```python
from build123d import *

# Parameters (mm, degrees)
SKETCH1_W           = 45
SKETCH1_H           = 37.5
BOSS_EXTRUDE1_DEPTH = 2
SKETCH2_W           = 40
SKETCH2_H           = 13
BOSS_EXTRUDE2_DEPTH = 7
BOSS_EXTRUDE3_DEPTH = 15
FILLET1_R           = 1
SKETCH4_W           = 10
SKETCH4_H           = 8
CUT_EXTRUDE1_DEPTH  = 5
SKETCH5_W           = 41
SKETCH5_H           = 14
CUT_EXTRUDE2_DEPTH  = 7
SKETCH6_W           = 11
SKETCH6_H           = 20
BOSS_EXTRUDE5_DEPTH = 12
SKETCH7_W           = 9
SKETCH7_H           = 9
CUT_EXTRUDE3_DEPTH  = 12


with BuildPart() as part:
    # Sketch1 → Boss-Extrude1 (new body)
    with BuildSketch(Plane.XY):
        Rectangle(SKETCH1_W, SKETCH1_H)
    extrude(amount=BOSS_EXTRUDE1_DEPTH)

    # Sketch2 → Boss-Extrude2 (add)
    with BuildSketch(Plane.XY.offset(2)):
        with Locations((0, -11.25)):
            Rectangle(SKETCH2_W, SKETCH2_H)
    extrude(amount=BOSS_EXTRUDE2_DEPTH)

    # Sketch3 → Boss-Extrude3 (add)
    with BuildSketch(Plane.XY.offset(9)):
        Polygon((-5, -7.25), (-5, -5.25), (-15, -5.25), (-15, -17.25), (-5, -17.25), (-5, -15.25), (5, -15.25), (5, -17.25), (15, -17.25), (15, -5.25), (5, -5.25), (5, -7.25), align=None)
    extrude(amount=BOSS_EXTRUDE3_DEPTH)

    # Fillet1
    fillet1_edges = [part.edges().sort_by_distance(p)[0] for p in [
        (5, -5.25, 16.5),
        (-5, -5.25, 16.5),
        (-15, -5.25, 16.5),
        (-15, -17.25, 16.5),
        (-5, -17.25, 16.5),
        (5, -17.25, 16.5),
        (15, -17.25, 16.5),
        (15, -5.25, 16.5),
    ]]
    fillet(fillet1_edges, radius=FILLET1_R)

    # Sketch4 → Cut-Extrude1 (cut)
    with BuildSketch(Plane.XY.offset(24)):
        with BuildLine():
            Line((-5.5, -14.75), (-5.5, -7.75))
            Line((-5.5, -7.75), (-5.5, -6.25))
            ThreePointArc((-5.5, -6.25), (-5.646446609, -5.896446609), (-6, -5.75))
            Line((-6, -5.75), (-14, -5.75))
            ThreePointArc((-14, -5.75), (-14.353553391, -5.896446609), (-14.5, -6.25))
            Line((-14.5, -6.25), (-14.5, -16.25))
            ThreePointArc((-14.5, -16.25), (-14.353553391, -16.603553391), (-14, -16.75))
            Line((-14, -16.75), (-6, -16.75))
            ThreePointArc((-6, -16.75), (-5.646446609, -16.603553391), (-5.5, -16.25))
            Line((-5.5, -16.25), (-5.5, -14.75))
        make_face()
        with BuildLine():
            Line((5.5, -7.75), (5.5, -14.75))
            Line((5.5, -14.75), (5.5, -16.25))
            ThreePointArc((5.5, -16.25), (5.646446609, -16.603553391), (6, -16.75))
            Line((6, -16.75), (14, -16.75))
            ThreePointArc((14, -16.75), (14.353553391, -16.603553391), (14.5, -16.25))
            Line((14.5, -16.25), (14.5, -6.25))
            ThreePointArc((14.5, -6.25), (14.353553391, -5.896446609), (14, -5.75))
            Line((14, -5.75), (6, -5.75))
            ThreePointArc((6, -5.75), (5.646446609, -5.896446609), (5.5, -6.25))
            Line((5.5, -6.25), (5.5, -7.75))
        make_face()
        with Locations((0, -11.25)):
            Rectangle(SKETCH4_W, SKETCH4_H)
    extrude(amount=-CUT_EXTRUDE1_DEPTH, mode=Mode.SUBTRACT)

    # Sketch5 → Cut-Extrude2 (cut)
    with BuildSketch(Plane.XY.offset(9)):
        with Locations((0, -11.25)):
            Rectangle(SKETCH5_W, SKETCH5_H)
        with BuildLine():
            Line((-14, -17.75), (-6, -17.75))
            ThreePointArc((-6, -17.75), (-4.939339828, -17.310660172), (-4.5, -16.25))
            Line((-4.5, -16.25), (-4.5, -15.75))
            Line((-4.5, -15.75), (4.5, -15.75))
            Line((4.5, -15.75), (4.5, -16.25))
            ThreePointArc((4.5, -16.25), (4.939339828, -17.310660172), (6, -17.75))
            Line((6, -17.75), (14, -17.75))
            ThreePointArc((14, -17.75), (15.060660172, -17.310660172), (15.5, -16.25))
            Line((15.5, -16.25), (15.5, -13.75))
            Line((15.5, -13.75), (17.5, -13.75))
            ThreePointArc((17.5, -13.75), (20, -11.25), (17.5, -8.75))
            Line((17.5, -8.75), (15.5, -8.75))
            Line((15.5, -8.75), (15.5, -6.25))
            ThreePointArc((15.5, -6.25), (15.060660172, -5.189339828), (14, -4.75))
            Line((14, -4.75), (6, -4.75))
            ThreePointArc((6, -4.75), (4.939339828, -5.189339828), (4.5, -6.25))
            Line((4.5, -6.25), (4.5, -6.75))
            Line((4.5, -6.75), (-4.5, -6.75))
            Line((-4.5, -6.75), (-4.5, -6.25))
            ThreePointArc((-4.5, -6.25), (-4.939339828, -5.189339828), (-6, -4.75))
            Line((-6, -4.75), (-14, -4.75))
            ThreePointArc((-14, -4.75), (-15.060660172, -5.189339828), (-15.5, -6.25))
            Line((-15.5, -6.25), (-15.5, -8.75))
            Line((-15.5, -8.75), (-17.5, -8.75))
            ThreePointArc((-17.5, -8.75), (-20, -11.25), (-17.5, -13.75))
            Line((-17.5, -13.75), (-15.5, -13.75))
            Line((-15.5, -13.75), (-15.5, -16.25))
            ThreePointArc((-15.5, -16.25), (-15.060660172, -17.310660172), (-14, -17.75))
        make_face(mode=Mode.SUBTRACT)
    extrude(amount=-CUT_EXTRUDE2_DEPTH, mode=Mode.SUBTRACT)

    # Sketch6 → Boss-Extrude5 (add)
    with BuildSketch(Plane(origin=(0, 0, 0), x_dir=(-1, 0, 0), z_dir=(0, 0, -1))):
        with Locations((-6, 8.25)):
            Rectangle(SKETCH6_W, SKETCH6_H)
        with Locations((6, 8.25)):
            Rectangle(SKETCH6_W, SKETCH6_H)
    extrude(amount=BOSS_EXTRUDE5_DEPTH)

    # Sketch7 → Cut-Extrude3 (cut)
    with BuildSketch(Plane(origin=(0, 18.25, 0), x_dir=(1, 0, 0), z_dir=(0, 1, 0))):
        with Locations((-6, 5.5)):
            Rectangle(SKETCH7_W, SKETCH7_H)
        with Locations((6, 5.5)):
            Rectangle(SKETCH7_W, SKETCH7_H)
    extrude(amount=-CUT_EXTRUDE3_DEPTH, mode=Mode.SUBTRACT)


solid = part.part
```
CAD build for the part. Positions are in the model's coordinates, mm. A direction names the side the tool comes from. Round coordinates to 2 decimals unless told otherwise and drop trailing zeros. Order: outer loops, then holes, each group sorted by start corner. A loop starts at its lowest first (then second) coordinate and runs counter-clockwise, first axis right, second up.
Q1. Slice it at B-B (z = 11.5). Write the cut outline in (x, y), and give its area (3 significant figures).
Q2. Wall check: L1, parallel to X at y = 10.5, z = -3.5; L2, parallel to X at y = -16, z = 10.5; L3, parallel to Z at x = 1, y = 5.5. Give the ranges that are in metal, low to high.
Q3. Which spindle directions (+Z, -Z, +X, -X, +Y, -Y) get a long thin tool onto all of the face, cutting with end or side? Do faces 1 (the cylindrical face through (-15.05, -5.18, 5.55)), 2 (the flat face through (-1, 18.25, -6)), 3 (the flat face through (15.5, -8, 6)), 4 (the cylindrical face through (15.05, -17.32, 5.55)), 5 (the flat face through (10, -16.75, 22)). Say none if no direction does.
Q4. Slice it at C-C (x = -9). Write the cut outline in (y, z), and give its area (3 significant figures).
Q5. Slice it at D-D (z = -2). Write the cut outline in (x, y).
Q6. Slice it at A-A (y = 8). Write the cut outline in (x, z).
Q7. Two-plate mould, pull along Z, no slides. Class faces 6 (the flat face through (10.5, 12, -5)), 7 (the flat face through (-10, -5.25, 16)), 8 (the flat face through (0, -11, 19)): pulls with the +Z half, pulls with the -Z half, needs draft (parallel to the pull), parting line crosses it, or undercut.
Q8. Drop flat-ended pins along their axis: pin 1 (10 mm diameter, centred on x = 6, y = 14.5, fed in from +Z); pin 2 (0.8 mm diameter, centred on y = -15.5, z = 5.5, fed in from +X); pin 3 (8 mm diameter, centred on y = -10.5, z = 17, fed in from +X). Give the stop position or say it passes through.
Results below:
1. outline: (-15, -16.25) arc R1 ccw to (-14, -17.25) - (-6, -17.25) arc R1 ccw to (-5, -16.25) - (-5, -15.25) - (5, -15.25) - (5, -16.25) arc R1 ccw to (6, -17.25) - (14, -17.25) arc R1 ccw to (15, -16.25) - (15, -6.25) arc R1 ccw to (14, -5.25) - (6, -5.25) arc R1 ccw to (5, -6.25) - (5, -7.25) - (-5, -7.25) - (-5, -6.25) arc R1 ccw to (-6, -5.25) - (-14, -5.25) arc R1 ccw to (-15, -6.25) - close
1. area: 318 mm2
2. L1: x = -11.5 to -10.5, -1.5 to -0.5, 0.5 to 1.5, 10.5 to 11.5
2. L2: x = -15 to -5, 5 to 15
2. L3: z = -12 to 2
3. face 1: +Z, -X, +Y
3. face 2: -Z, +X, -X, +Y
3. face 3: +Z, +X, +Y
3. face 4: +Z, +X, -Y
3. face 5: +Z
4. outline: (-18.75, 0) - (-1.75, 0) - (-1.75, -12) - (18.25, -12) - (18.25, -10) - (6.25, -10) - (6.25, -1) - (18.25, -1) - (18.25, 0) - (18.75, 0) - (18.75, 2) - (-4.75, 2) - (-4.75, 9) - (-5.25, 9) - (-5.25, 24) - (-5.75, 24) - (-5.75, 19) - (-16.75, 19) - (-16.75, 24) - (-17.25, 24) - (-17.25, 9) - (-17.75, 9) - (-17.75, 2) - (-18.75, 2) - close
4. area: 423 mm2
5. outline: (-11.5, -1.75) - (-0.5, -1.75) - (-0.5, 18.25) - (-1.5, 18.25) - (-1.5, 6.25) - (-10.5, 6.25) - (-10.5, 18.25) - (-11.5, 18.25) - close; (0.5, -1.75) - (11.5, -1.75) - (11.5, 18.25) - (10.5, 18.25) - (10.5, 6.25) - (1.5, 6.25) - (1.5, 18.25) - (0.5, 18.25) - close
6. outline: (-22.5, 0) - (-11.5, 0) - (-11.5, -12) - (-0.5, -12) - (-0.5, 0) - (0.5, 0) - (0.5, -12) - (11.5, -12) - (11.5, 0) - (22.5, 0) - (22.5, 2) - (-22.5, 2) - close; hole (-10.5, -10) - (-1.5, -10) - (-1.5, -1) - (-10.5, -1) - close; hole (1.5, -10) - (10.5, -10) - (10.5, -1) - (1.5, -1) - close
7. face 6: undercut
7. face 7: needs draft
7. face 8: pulls with the +Z half
8. pin 1: stops at z = 2
8. pin 2: stops at x = 15.5
8. pin 3: stops at x = 15
